```python
from build123d import *

# Parameters (mm, degrees)
SKETCH002_R       = 1.5
SKETCH002_R_2     = 3
PAD_DEPTH         = 5
SKETCH003_W       = 14
SKETCH003_H       = 22.5
PAD001_DEPTH      = 63
SKETCH004_W       = 4.24264
SKETCH004_H       = 4.24264
PAD002_DEPTH      = 5
SKETCH005_R       = 1.5
SKETCH005_R_2     = 3
PAD003_DEPTH      = 5
SKETCH006_R       = 4
POCKET_DEPTH      = 21.777567
POCKET_DEPTH_BACK = 7.001


with BuildPart() as part:
    # Sketch002 → Pad (new body)
    with BuildSketch(Plane.XY):
        with BuildLine():
            ThreePointArc((7, 63.652914), (5.369142, 68.007903), (1.278873, 70.220442))
            ThreePointArc((1.278873, 70.220442), (-17.873705, 64.296837), (-19.425905, 44.309315))
            ThreePointArc((-19.425905, 44.309315), (-16.29285, 41.155365), (-12, 40))
            ThreePointArc((-7, 35), (-8.464466, 38.535534), (-12, 40))
            Line((-7, 35), (-7, 0))
            ThreePointArc((-7, 0), (0, -7), (7, 0))
            Line((7, 0), (7, 63.652914))
        make_face()
        with Locations((-16.5, 53)):
            Circle(SKETCH002_R, mode=Mode.SUBTRACT)
        with Locations((-4.5, 53)):
            Circle(SKETCH002_R_2, mode=Mode.SUBTRACT)
        with Locations((-4.5, 65)):
            Circle(SKETCH002_R, mode=Mode.SUBTRACT)
        Circle(SKETCH002_R_2, mode=Mode.SUBTRACT)
    extrude(amount=PAD_DEPTH)

    # Sketch003 → Pad001 (join)
    with BuildSketch(Plane.XY):
        with Locations((0, 23.75)):
            Rectangle(SKETCH003_W, SKETCH003_H)
    extrude(amount=-PAD001_DEPTH)

    # Sketch004 (on DatumPlane) → Pad002 (join)
    with BuildSketch(Plane.XY.offset(-63)):
        with BuildLine():
            ThreePointArc((-7, 0), (0, -7), (7, 0))
            Line((7, 0), (7, 35))
            Line((7, 35), (-7, 35))
            Line((-7, 35), (-7, 0))
        make_face()
        Rectangle(SKETCH004_W, SKETCH004_H, mode=Mode.SUBTRACT)
    extrude(amount=-PAD002_DEPTH)

    # Sketch005 → Pad003 (join)
    with BuildSketch(Plane.XY.offset(-16)):
        with BuildLine():
            Line((-7, 35), (7, 35))
            Line((7, 35), (7, 63.652914))
            ThreePointArc((7, 63.652914), (5.369142, 68.007903), (1.278873, 70.220442))
            ThreePointArc((1.278873, 70.220442), (-17.873705, 64.296837), (-19.425905, 44.309315))
            ThreePointArc((-19.425905, 44.309315), (-16.29285, 41.155365), (-12, 40))
            ThreePointArc((-7, 35), (-8.464466, 38.535534), (-12, 40))
        make_face()
        with Locations((-16.5, 53)):
            Circle(SKETCH005_R, mode=Mode.SUBTRACT)
        with Locations((-4.5, 53)):
            Circle(SKETCH005_R_2, mode=Mode.SUBTRACT)
        with Locations((-4.5, 65)):
            Circle(SKETCH005_R, mode=Mode.SUBTRACT)
    extrude(amount=-PAD003_DEPTH)

    # Sketch006 → Pocket (cut, two sides)
    with BuildSketch(Plane.YZ) as pocket_sk:
        with Locations((22.75, -8)):
            Circle(SKETCH006_R)
        with Locations((22.75, -28)):
            Circle(SKETCH006_R)
    extrude(amount=-POCKET_DEPTH, mode=Mode.SUBTRACT)
    extrude(pocket_sk.sketch, amount=POCKET_DEPTH_BACK, mode=Mode.SUBTRACT)


with BuildPart() as part_1:
    # Body placement: moved
    add(part.part.moved(Location((0, 0, -5))))


solid = part_1.part
```
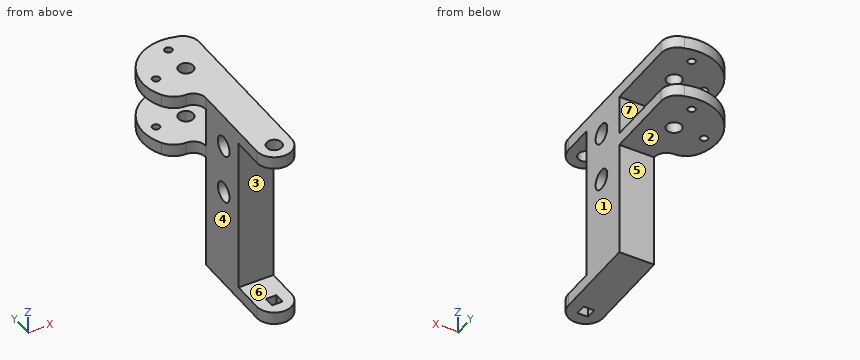
For this review, take the finished solid that the model builds, in its own axes (mm). Face numbers are marked on the shaded views. A direction names the side the tool comes from. Round coordinates to 2 decimals unless told otherwise and drop trailing zeros. Write each loop counter-clockwise with the first axis right and the second up, starting at its lowest first coordinate (ties: lowest second). Pieces come first, ordered by that corner, then holes. Notation, with made-up numbers: (-36.75, 60.25) -> (13.25, 60.25) arc R20 ccw to (13.25, 78.25) -> close; hole circle Ø7 at (61, -6.5). An arc over 180 degrees is marked (long way). One line per question, with ' | ' between items. Start each with the question number.
1) Mouldability with a two-part tool opening along Z and no side actions: class the marked faces 1, 2 and 3 as +Z half, -Z half, draft (parallel to the pull), parting line (faces both ways), or undercut.
2) Add section D-D (y = 8.5). Write out the cut boundary in (x, z).
3) Add section A-A (y = 22.75). Write out the cut boundary in (x, z), and give its area (3 significant figures).
4) Add section C-C (z = -13). Write out the cut boundary in (x, y), and give its area (3 significant figures).
5) Wall thickness on line 1 along Y through (x, z) = (-4.5, -24.65); line 2 along Z through (x, y) = (4, 22.75); line 3 along Z through (x, y) = (-15.5, 57): over which ranges is each line inside the solid? List them lowest first.
6) For pin 1 Ø4 at (x, y) = (2.5, 7) entering from +Z; pin 2 Ø12 at (x, z) = (-8.5, -37.5) entering from -Y; pin 3 Ø8.5 at (x, y) = (-13, 60) entering from -Z; pin 4 Ø8 at (y, z) = (12, -34.5) entering from -X, all flat-tipped, find the tip position at first contact; note any pin that passes through.
7) Machinability: for the marked faces 4, 5, 6 and 7, which of the approach directions +Z, -Z, +X, -X, +Y, -Y give a long, thin tool a straight path to every point of the face, cutting with its end or side? Answer none if there is none.
8) Add section B-B (x = 0). Write out the cut boundary in (y, z), and give its area (3 significant figures).
Reported:
1) face 1: draft | face 2: -Z half | face 3: undercut
2) outline: (-7, -73) -> (7, -73) -> (7, -68) -> (-7, -68) -> close; (-7, -5) -> (7, -5) -> (7, 0) -> (-7, 0) -> close
3) outline: (-7, -73) -> (7, -73) -> (7, -37) -> (-7, -37) -> close; (-7, -29) -> (7, -29) -> (7, -17) -> (-7, -17) -> close; (-7, -9) -> (7, -9) -> (7, 0) -> (-7, 0) -> close | area: 798 mm²
4) outline: (-7, 12.5) -> (7, 12.5) -> (7, 18.75) -> (-7, 18.75) -> close; (-7, 26.75) -> (7, 26.75) -> (7, 35) -> (-7, 35) -> close | area: 203 mm²
5) line 1: y = 12.5 to 50, 56 to 63.5, 66.5 to 70.99 | line 2: z = -73 to -37, -29 to -17, -9 to 0 | line 3: z = -26 to -21, -5 to 0
6) pin 1: stops at z = 0 | pin 2: stops at y = 12.5 | pin 3: stops at z = -26 | pin 4: stops at x = -7
7) face 4: +Z, -Z, -X, -Y | face 5: -Z, +X, -X, +Y | face 6: +X, -X, -Y | face 7: +X, -X, +Y
8) outline: (-7, -73) -> (-2.12, -73) -> (-2.12, -68) -> (-7, -68) -> close; (-7, -5) -> (-3, -5) -> (-3, 0) -> (-7, 0) -> close; (2.12, -73) -> (35, -73) -> (35, -26) -> (70.56, -26) -> (70.56, -21) -> (35, -21) -> (35, -5) -> (70.56, -5) -> (70.56, 0) -> (3, 0) -> (3, -5) -> (12.5, -5) -> (12.5, -68) -> (2.12, -68) -> close; hole circle Ø8 at (22.75, -33); hole circle Ø8 at (22.75, -13) | area: 2,040 mm²
